from build123d import *

# Parameters (mm, degrees)
PAD001_DEPTH = 0.2
PAD002_DEPTH = 5.08
FILLET_R     = 0.5
SKETCH_R     = 0.225
PAD_DEPTH    = 3


with BuildPart() as pad001:
    # Sketch001 → Pad001 (new body)
    with BuildSketch(Plane.XY.offset(0.8)):
        with BuildLine():
            Line((-2.645, -2.475), (16.655, -2.475))
            ThreePointArc((16.655, -2.475), (17.362107, -2.182107), (17.655, -1.475))
            Line((17.655, -1.475), (17.655, 9.225))
            ThreePointArc((17.655, 9.225), (17.362107, 9.932107), (16.655, 10.225))
            Line((16.655, 10.225), (-1.645, 10.225))
            ThreePointArc((-1.645, 10.225), (-2.352107, 9.932107), (-2.645, 9.225))
            Line((-2.645, 9.225), (-2.645, -2.475))
        make_face()
    extrude(amount=PAD001_DEPTH)


with BuildPart() as fillet_body:
    # Sketch002 → Pad002 (new body)
    with BuildSketch(Plane.XY.offset(0.8)):
        with BuildLine():
            Line((-1.465, -1.975), (16.835, -1.975))
            ThreePointArc((16.835, -1.975), (17.188553, -1.828553), (17.335, -1.475))
            Line((17.335, -1.475), (17.335, 9.225))
            ThreePointArc((17.335, 9.225), (17.188553, 9.578553), (16.835, 9.725))
            Line((16.835, 9.725), (-1.465, 9.725))
            ThreePointArc((-1.465, 9.725), (-1.818553, 9.578553), (-1.965, 9.225))
            Line((-1.965, 9.225), (-1.965, -1.475))
            ThreePointArc((-1.965, -1.475), (-1.818553, -1.828553), (-1.465, -1.975))
        make_face()
    extrude(amount=PAD002_DEPTH)

    # Fillet
    fillet_edges = [fillet_body.edges().sort_by_distance(p)[0] for p in [
        (-1.818553, -1.828553, 5.88),
        (7.685, -1.975, 5.88),
        (-1.965, 3.875, 5.88),
        (-1.818553, 9.578553, 5.88),
        (7.685, 9.725, 5.88),
        (17.188553, 9.578553, 5.88),
        (17.335, 3.875, 5.88),
        (17.188553, -1.828553, 5.88),
    ]]
    fillet(fillet_edges, radius=FILLET_R)


with BuildPart() as obj1:
    # Sketch → Pad (new body)
    with BuildSketch(Plane.XY.offset(0.8)):
        Circle(SKETCH_R)
        with Locations((15.37, 0)):
            Circle(SKETCH_R)
        with Locations((15.37, 7.75)):
            Circle(SKETCH_R)
        with Locations((0, 7.75)):
            Circle(SKETCH_R)
    extrude(amount=-PAD_DEPTH)

    # obj1: union Pad001, Fillet body
    add(pad001.part)
    add(fillet_body.part)


solid = obj1.part
Input: part model. Units: mm. Frame: model coordinates. A direction names the side the tool comes from. Round coordinates to 2 decimals unless told otherwise and drop trailing zeros. Order: outer loops, then holes, each group sorted by start corner. A loop starts at its lowest first (then second) coordinate and runs counter-clockwise, first axis right, second up. Notation, with made-up numbers: (-28, 36) - (-7, 36) arc R20 cw to (-7, 48) - close; hole circle Ø11 at (-15.75, -4.75). An arc over 180 degrees is marked (long way). Answer as a JSON object with one key per item and string values. Group by question number.
(1) Cut plane A-A (z = 2.5). Return loops of the section in (x, y) (3 decimals).
(2) Material intervals for probe 1 along Z at (x, y) = (0.5, 5); probe 2 along X at (y, z) = (4.5, 1.5) (3 decimals); probe 3 along Y at (x, z) = (13, 4.5) (3 decimals), sorted ascending. Write a range as from..to.
(3) Draft query along X for faces 1 (the face through (-1.965, 4, 3)), 2 (the face through (8, 9.725, 3)), 3 (the face through (17.335, 4, 3)). Return one class per face: released by +X, released by -X, zero draft, split by the parting line, or undercut.
(4) Cut plane C-C (z = 0.5). Return loops of the section in (x, y) (3 decimals).
(5) Cut plane D-D (x = 8.25). Return loops of the section in (y, z) (3 decimals).
(6) Reachability of faces 4 (the face through (8, -1.975, 3)), 5 (the face through (8, 4, 5.88)) from +Z, -Z, +X, -X, +Y, -Y: full face, straight path, thin tool, end or side. Return the list, or none.
(7) Pin query (flat end, axial travel): P1, Ø1.3, axis at y = 3, z = 3.5, coming from the -X side (3 decimals); P2, Ø2, axis at y = 4, z = 4, coming from the +X side (3 decimals); P3, Ø3.5, axis at x = 6.5, z = 3, coming from the +Y side (3 decimals). Return the tip coordinate at first contact, or that it passes through.
(8) Cut plane B-B (y = 7.75). Return loops of the section in (x, z) (3 decimals).
Here are the results:
{
 "1": {"outline": "(-1.965, -1.475) arc R0.5 ccw to (-1.465, -1.975) - (16.835, -1.975) arc R0.5 ccw to (17.335, -1.475) - (17.335, 9.225) arc R0.5 ccw to (16.835, 9.725) - (-1.465, 9.725) arc R0.5 ccw to (-1.965, 9.225) - close"},
 "2": {"probe 1": "z = 0.8..5.88", "probe 2": "x = -1.965..17.335", "probe 3": "y = -1.975..9.725"},
 "3": {"face 1": "released by -X", "face 2": "zero draft", "face 3": "released by +X"},
 "4": {"outline": "circle Ø0.45 at (0, 0); circle Ø0.45 at (0, 7.75); circle Ø0.45 at (15.37, 0); circle Ø0.45 at (15.37, 7.75)"},
 "5": {"outline": "(-2.475, 0.8) - (10.225, 0.8) - (10.225, 1) - (9.725, 1) - (9.725, 5.38) arc R0.5 ccw to (9.225, 5.88) - (-1.475, 5.88) arc R0.5 ccw to (-1.975, 5.38) - (-1.975, 1) - (-2.475, 1) - close"},
 "6": {"face 4": "+Z, +X, -X, -Y", "face 5": "+Z, +X, -X, +Y, -Y"},
 "7": {"P1": "stops at x = -1.965", "P2": "stops at x = 17.335", "P3": "stops at y = 9.725"},
 "8": {"outline": "(-2.645, 0.8) - (-0.225, 0.8) - (-0.225, -2.2) - (0.225, -2.2) - (0.225, 0.8) - (15.145, 0.8) - (15.145, -2.2) - (15.595, -2.2) - (15.595, 0.8) - (17.655, 0.8) - (17.655, 1) - (17.335, 1) - (17.335, 5.38) arc R0.5 ccw to (16.835, 5.88) - (-1.465, 5.88) arc R0.5 ccw to (-1.965, 5.38) - (-1.965, 1) - (-2.645, 1) - close"}
}
